from build123d import *

# Parameters (mm, degrees)
SKETCH1_W             = 84.5
SKETCH1_H             = 62
PCB_DEPTH             = 1.6
SKETCH2_W             = 9.5
SKETCH2_H             = 31
TERMINAL_BLOCK_DEPTH  = 10.9
SKETCH3_W             = 9.5
SKETCH3_H             = 31
TERMINAL_PINS_DEPTH   = 2.5
SKETCH4_W             = 63
SKETCH4_H             = 56
COMPONENTS_DEPTH      = 4.4
SKETCH5_W             = 20
SKETCH5_H             = 14
INPUT_CONNECTOR_DEPTH = 7.4
SKETCH6_R             = 5.3
CAP_1_DEPTH           = 11
SKETCH7_R             = 5.3
CAP_2_DEPTH           = 11


with BuildPart() as part:
    # Sketch1 → PCB (new body)
    with BuildSketch(Plane.XY):
        Rectangle(SKETCH1_W, SKETCH1_H)
    extrude(amount=PCB_DEPTH)

    # Sketch2 → Terminal_block (add)
    with BuildSketch(Plane.XY.offset(1.6)):
        with Locations((-33.75, 0)):
            Rectangle(SKETCH2_W, SKETCH2_H)
    extrude(amount=TERMINAL_BLOCK_DEPTH)

    # Sketch3 → Terminal_pins (add)
    with BuildSketch(Plane.XY.offset(-2.5)):
        with Locations((-33.75, 0)):
            Rectangle(SKETCH3_W, SKETCH3_H)
    extrude(amount=TERMINAL_PINS_DEPTH)

    # Sketch4 → Components (add)
    with BuildSketch(Plane.XY.offset(1.6)):
        with Locations((2.5, 0)):
            Rectangle(SKETCH4_W, SKETCH4_H)
    extrude(amount=COMPONENTS_DEPTH)

    # Sketch5 → Input_connector (add)
    with BuildSketch(Plane.XY.offset(1.6)):
        with Locations((44, 0)):
            Rectangle(SKETCH5_W, SKETCH5_H)
    extrude(amount=INPUT_CONNECTOR_DEPTH)

    # Sketch6 → Cap_1 (add)
    with BuildSketch(Plane.XY.offset(1.6)):
        with Locations(Location((-25.3, 1.2, 0), (0, 0, 225.724178288))):
            Circle(SKETCH6_R)
    extrude(amount=CAP_1_DEPTH)

    # Sketch7 → Cap_2 (add)
    with BuildSketch(Plane.XY.offset(1.6)):
        with Locations((-10, 1.2)):
            Circle(SKETCH7_R)
    extrude(amount=CAP_2_DEPTH)


solid = part.part
Verification items for the finished model (mm, model axes). A direction names the side the tool comes from. Coordinates: 2 decimals unless noted, no trailing zeros. Loops run counter-clockwise (first coordinate to the right, second up) from the corner with the lowest first, then second, coordinate; pieces in that order, holes last. Notation, with made-up numbers: (23, -33.75) -> (79, -33.75) arc R19 ccw to (79, -14.75) -> close; hole circle Ø1 at (-3, 10). An arc over 180 degrees is marked (long way). Write each question's results on one line, items separated by ' | '.
Item 1: Material ranges on L1, parallel to Z at x = -31, y = -7; L2, parallel to Z at x = 40.5, y = -3.5; L3, parallel to Y at x = 7, z = 4.75, recorded low to high.
Found:
L1: z = -2.5 to 12.5 | L2: z = 0 to 9 | L3: y = -28 to 28
Item 2: Mould release check, pull along X, two halves, no side actions. Record for faces 4 (the face through (-38.5, 0, -1)), 5 (the face through (-29, 0, -1)), 6 (the face through (-29, -9, 9)): +X half, -X half, draft (parallel to the pull), parting line (faces both ways), or undercut.
Found:
face 4: -X half | face 5: +X half | face 6: undercut
Item 3: Section check A-A, the plane x = -17. Enter the section's corners in (y, z).
Found:
outline: (-31, 0) -> (31, 0) -> (31, 1.6) -> (28, 1.6) -> (28, 6) -> (-28, 6) -> (-28, 1.6) -> (-31, 1.6) -> close
Item 4: Section check D-D, the plane y = -9.5. Enter the section's corners in (x, z), plus the area to 3 significant figures.
Found:
outline: (-42.25, 0) -> (-38.5, 0) -> (-38.5, -2.5) -> (-29, -2.5) -> (-29, 0) -> (42.25, 0) -> (42.25, 1.6) -> (34, 1.6) -> (34, 6) -> (-29, 6) -> (-29, 12.5) -> (-38.5, 12.5) -> (-38.5, 1.6) -> (-42.25, 1.6) -> close | area: 540 mm2
Item 5: Section check B-B, the plane y = -17. Enter the section's corners in (x, z), plus the area to 3 significant figures.
Found:
outline: (-42.25, 0) -> (42.25, 0) -> (42.25, 1.6) -> (34, 1.6) -> (34, 6) -> (-29, 6) -> (-29, 1.6) -> (-42.25, 1.6) -> close | area: 412 mm2
Item 6: Section check C-C, the plane z = 4.5. Enter the section's corners in (x, y), plus the area to 3 significant figures.
Found:
outline: (-38.5, -15.5) -> (-29, -15.5) -> (-29, -28) -> (34, -28) -> (34, -7) -> (54, -7) -> (54, 7) -> (34, 7) -> (34, 28) -> (-29, 28) -> (-29, 15.5) -> (-38.5, 15.5) -> close | area: 4,100 mm2
Item 7: Tool access check on faces 1 (the face through (34, 17, 4)), 2 (the face through (2, 0, 6)), 3 (the face through (-34, -15.5, -1)). Record the directions out of +Z, -Z, +X, -X, +Y, -Y that give a thin tool (end or side, any length) a straight path to the whole face; none if there is none.
Found:
face 1: +Z, +X, +Y | face 2: +Z | face 3: -Z, +X, -X, -Y
Item 8: Gauge pin test, flat ends, axial feed: pin 1 (2 mm diameter, centred on x = -36, z = -1.5, fed in from -Y); pin 2 (1.2 mm diameter, centred on y = 0, z = -1, fed in from -X); pin 3 (12 mm diameter, centred on x = -14.5, y = -16, fed in from +Z). Record the tip position at first contact, or that the pin passes through.
Found:
pin 1: stops at y = -15.5 | pin 2: stops at x = -38.5 | pin 3: stops at z = 6
